from build123d import *

# Parameters (mm, degrees)
F0_R     = 30.3
F1_DEPTH = 14
F2_R     = 28.8
F3_DEPTH = 13
F4_R     = 4
F5_DEPTH = 25.4
F6_R     = 0.99999


# Not quite as in the source:
# - a fillet or chamfer is up to 0.001 mm smaller than in the source, because OpenCascade refuses the exact size


with BuildPart() as f1:
    # F0 (on Top) → F1 (new body)
    with BuildSketch(Plane.XY):
        Circle(F0_R)
    extrude(amount=F1_DEPTH)

    # F2 (on face) → F3 (cut)
    with BuildSketch(Plane.XY.offset(14)):
        Circle(F2_R)
    extrude(amount=-F3_DEPTH, mode=Mode.SUBTRACT)

    # F4 (on face) → F5 (cut)
    with BuildSketch(Plane.XY.offset(1)):
        Circle(F4_R)
    extrude(amount=-F5_DEPTH, mode=Mode.SUBTRACT)

    # F6 (radius 1 in the source; OpenCascade refuses exactly that, so slightly less here)
    f6_edges = [f1.edges().sort_by_distance(p)[0] for p in [
        (-30.3, 0, 0),
        (-4, 0, 0),
        (-30.3, 0, 14),
    ]]
    fillet(f6_edges, radius=F6_R)


solid = f1.part
Read the model definition and answer for the solid it produces. Units are mm, in the model's axes. Coordinates: 2 decimals unless noted, no trailing zeros. Write each loop counter-clockwise with the first axis right and the second up, starting at its lowest first coordinate (ties: lowest second). Pieces come first, ordered by that corner, then holes. Notation, with made-up numbers: M 21.5,-26 L 77.5,-26 A31 ccw 77.5,10 Z; hole C 88,-24.75 d8. An arc over 180 degrees is marked long. Use a Markdown table: item, result.
Q1. Each of these flat-tipped pins is pushed along its axis until it touches: pin 1 Ø4 at (x, y) = (-18, 5.5) entering from +Z; pin 2 Ø5 at (x, z) = (-8.5, 12.5) entering from -Y; pin 3 Ø6 at (y, z) = (8, 11) entering from -X. Where does it stop, or does it pass through?
Answer block:
| item | result |
|---|---|
| pin 1 | stops at z = 1 |
| pin 2 | stops at y = -29.7 |
| pin 3 | stops at x = -29.88 |
Q2. Straight lines are drawn through the part: L1, parallel to Y at x = 0, z = 1.05; L2, parallel to Z at x = -14.5, y = 5; L3, parallel to X at y = 7.5, z = 5.75. For each, find the intervals that lie inside material, in ascending order. Write a range as [from, to].
Answer block:
| item | result |
|---|---|
| L1 | y = [-30.3, -28.8], [28.8, 30.3] |
| L2 | z = [0, 1] |
| L3 | x = [-29.36, -27.81], [27.81, 29.36] |
Q3. The part is cut by section C-C, the plane z = 2.25. Write down the section's boundary in (x, y), then the cut area to 3 significant figures.
Answer block:
| item | result |
|---|---|
| outline | C 0,0 d60.6; hole C 0,0 d57.6 |
| area | 279 mm2 |
Q4. Determine the mould class of faces 1 (the face through (-24.045, -18.437, 6.916)), 2 (the face through (6, 0, 0)), 3 (the face through (0, -6, 1)), 4 (the face through (27.47, 8.65, 7.59)) for opening direction X: released by +X, released by -X, zero draft, split by the parting line, or undercut.
Answer block:
| item | result |
|---|---|
| face 1 | split by the parting line |
| face 2 | zero draft |
| face 3 | undercut |
| face 4 | undercut |
